Design review of the part shown in the three views and the two pictorial views. Dimensions are in mm from the part's minimum x, y and z. A direction names the side the tool comes from. Round coordinates to 2 decimals unless told otherwise and drop trailing zeros. Write each loop counter-clockwise with the first axis right and the second up, starting at its lowest first coordinate (ties: lowest second). Pieces come first, ordered by that corner, then holes. Notation, with made-up numbers: (33, -5.5) -> (61, -5.5) arc R33 cw to (61, 30.5) -> close; hole circle Ø3 at (40.25, -28.75). An arc over 180 degrees is marked (long way). Return JSON: item names as keys, results as strings. Group by question number.
1. Take a section at B-B, the plane y = 11. Write out the cut boundary in (x, z), then the cut area to 3 significant figures.
2. For line 1 along Y through (x, z) = (12.7, 2.9); line 2 along X through (y, z) = (17, 9) (1 decimal); line 3 along Z through (x, y) = (11.5, 3), list the stretches that pass through material, from the lowest coordinate up. Write a range as from..to.
3. Mouldability with a two-part tool opening along Z and no side actions: class the marked faces 1, 2, 3 and 4 as pulls with the +Z half, pulls with the -Z half, needs draft (parallel to the pull), parting line crosses it, or undercut.
4. Take a section at D-D, the plane x = 17.5. Write out the cut boundary in (y, z).
5. Clearance check with flat-ended pins moving along their axes: P1, Ø10, axis at x = 9, y = 9, coming from the -Z side; P2, Ø5.5, axis at y = 10.5, z = 14, coming from the -X side; P3, Ø1, axis at x = 10.5, z = 3.5, coming from the -Y side; P4, Ø8, axis at x = 22, z = 12, coming from the -Y side (1 decimal). State where each tip first meets the part, or that it passes through.
6. Take a section at C-C, the plane x = 21.5. Write out the cut boundary in (y, z) (1 decimal).
7. Take a section at A-A, the plane z = 11.75. Write out the cut boundary in (x, y).
8. Tool access review of the marked faces 5, 6, 7 and 8: name each direction out of +Z, -Z, +X, -X, +Y, -Y from which nothing blocks a thin tool from reaching the whole face with its end or side.
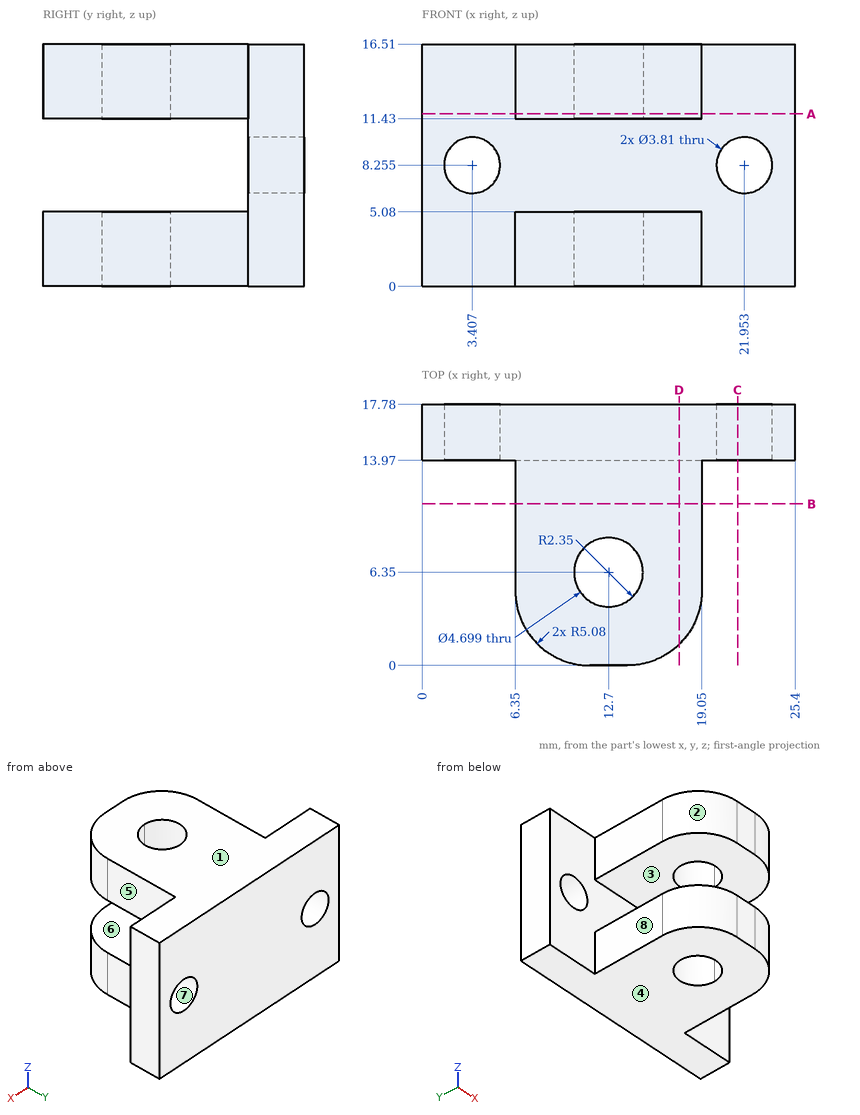
Output:
{
 "1": {"outline": "(6.35, 0) -> (19.05, 0) -> (19.05, 5.08) -> (6.35, 5.08) -> close; (6.35, 11.43) -> (19.05, 11.43) -> (19.05, 16.51) -> (6.35, 16.51) -> close", "area": "129 mm^2"},
 "2": {"line 1": "y = 0..4, 8.7..17.78", "line 2": "x = 0..1.7, 5.2..20.2, 23.7..25.4", "line 3": "z = 0..5.08, 11.43..16.51"},
 "3": {"face 1": "pulls with the +Z half", "face 2": "needs draft", "face 3": "undercut", "face 4": "pulls with the -Z half"},
 "4": {"outline": "(1.43, 0) -> (17.78, 0) -> (17.78, 16.51) -> (1.43, 16.51) -> (1.43, 11.43) -> (13.97, 11.43) -> (13.97, 5.08) -> (1.43, 5.08) -> close"},
 "5": {"P1": "stops at z = 0", "P2": "stops at x = 6.35", "P3": "stops at y = 0.02", "P4": "stops at y = 2"},
 "6": {"outline": "(14, 0) -> (17.8, 0) -> (17.8, 6.4) -> (14, 6.4) -> close; (14, 10.1) -> (17.8, 10.1) -> (17.8, 16.5) -> (14, 16.5) -> close"},
 "7": {"outline": "(0, 13.97) -> (6.35, 13.97) -> (6.35, 5.08) arc R5.08 ccw to (11.43, 0) -> (13.97, 0) arc R5.08 ccw to (19.05, 5.08) -> (19.05, 13.97) -> (25.4, 13.97) -> (25.4, 17.78) -> (0, 17.78) -> close; hole (12.7, 4) arc R2.35 ccw to (15.05, 6.35) arc R2.35 ccw (long way) to start"},
 "8": {"face 5": "+Z, -Z, +X, -Y", "face 6": "+X, -X, -Y", "face 7": "+Y, -Y", "face 8": "+Z, -Z, -X, -Y"}
}
